Model file for the job. Use its own axes, mm. Face numbers are marked on the shaded views. A direction names the side the tool comes from. Round coordinates to 2 decimals unless told otherwise and drop trailing zeros. Loops run counter-clockwise (first coordinate to the right, second up) from the corner with the lowest first, then second, coordinate; pieces in that order, holes last. Notation, with made-up numbers: M 3,55 L 25,55 A11 ccw 25,71 Z; hole C 34.5,2.5 d6. An arc over 180 degrees is marked long. Use a Markdown table: item, result. Add a question column.
Item 1: Two-plate mould, pull along Z, no slides. Class the marked faces 1, 2, 3 and 4: +Z half, -Z half, draft (parallel to the pull), parting line (faces both ways), or undercut.
Item 2: Pin check, flat tips, straight feed: P1, Ø0.8, axis at x = 14, z = 10.5, coming from the -Y side; P2, Ø10, axis at x = 24.5, y = -14.5, coming from the +Z side; P3, Ø12, axis at x = 4.5, z = 39.5, coming from the +Y side. Stop position of each tip, or through.
Item 3: Tool access for the marked faces 5, 6, 7 and 8: list every direction of +Z, -Z, +X, -X, +Y, -Y with a clear straight run to the whole face (end or side of a thin tool).
Item 4: Saw through at C-C on y = 29. Write the cut outline in (x, z).
Item 5: Saw through at D-D on z = 17.5. Write the cut outline in (x, y).
Item 6: Wall check: L1, parallel to Z at x = 26, y = 15; L2, parallel to X at y = 40, z = 59.7; L3, parallel to Z at x = 7.5, y = -40. Give the ranges that are in metal, low to high. Write a range as from..to.
Item 7: Saw through at A-A on y = -34. Write the cut outline in (x, z).
Item 8: Saw through at B-B on y = -46. Write the cut outline in (x, z).
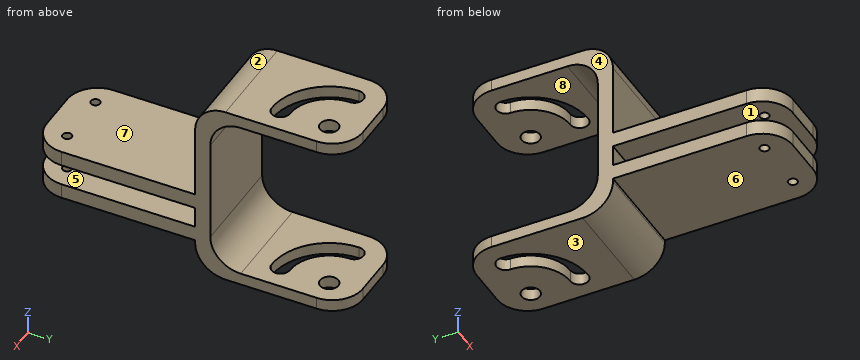
```python
from build123d import *

# Parameters (mm, degrees)
ESBO_O1_W                = 33
ESBO_O1_H                = 50
ESBO_O1_R                = 3
RESSALTO_EXTRUS_O2_DEPTH = 62
ESBO_O3_W                = 33
ESBO_O3_H                = 54
CORTE_EXTRUS_O1_DEPTH    = 45
ESBO_O7_W                = 33
ESBO_O7_H                = 5
RESSALTO_EXTRUS_O3_DEPTH = 54
ESBO_O10_R               = 1.5
CORTE_EXTRUS_O2_DEPTH    = 82.277303105
FILETE1_R                = 10


with BuildPart() as part:
    # Esboço1 → Ressalto-extrusão2 (new body)
    with BuildSketch(Plane.XY):
        with Locations((16.5, 25)):
            Rectangle(ESBO_O1_W, ESBO_O1_H)
        with Locations((25, 40)):
            Circle(ESBO_O1_R, mode=Mode.SUBTRACT)
        with BuildLine():
            ThreePointArc((6, 40), (11.564971157, 26.564971157), (25, 21))
            ThreePointArc((25, 21), (28, 24), (25, 27))
            ThreePointArc((25, 27), (15.807611845, 30.807611845), (12, 40))
            ThreePointArc((12, 40), (9, 43), (6, 40))
        make_face(mode=Mode.SUBTRACT)
    extrude(amount=RESSALTO_EXTRUS_O2_DEPTH)

    # Esboço3 → Corte-extrusão1 (cut)
    with BuildSketch(Plane(origin=(0, 50, 0), x_dir=(1, 0, 0), z_dir=(0, 1, 0))):
        with Locations((16.5, -31)):
            Rectangle(ESBO_O3_W, ESBO_O3_H)
    extrude(amount=-CORTE_EXTRUS_O1_DEPTH, mode=Mode.SUBTRACT)

    # Esboço7 → Ressalto-extrusão3 (add)
    with BuildSketch(Plane.XZ):
        with Locations((16.5, 25.5)):
            Rectangle(ESBO_O7_W, ESBO_O7_H)
        with Locations((16.5, 13.5)):
            Rectangle(ESBO_O7_W, ESBO_O7_H)
    extrude(amount=RESSALTO_EXTRUS_O3_DEPTH)

    # Esboço10 → Corte-extrusão2 (cut, through all)
    with BuildSketch(Plane(origin=(0, 0, 11), x_dir=(-1, 0, 0), z_dir=(0, 0, -1))):
        with Locations((-25.5, -46)):
            Circle(ESBO_O10_R)
        with Locations((-7.5, -46)):
            Circle(ESBO_O10_R)
    extrude(amount=-CORTE_EXTRUS_O2_DEPTH, mode=Mode.SUBTRACT)

    # Filete1
    filete1_edges = [part.edges().sort_by_distance(p)[0] for p in [
        (0, 50, 2),
        (33, 50, 2),
        (16.5, 5, 4),
        (16.5, 5, 58),
        (16.5, 0, 62),
        (16.5, 0, 0),
        (33, -54, 25.5),
        (0, -54, 25.5),
        (33, -54, 13.5),
        (0, -54, 13.5),
        (0, 50, 60),
        (33, 50, 60),
    ]]
    fillet(filete1_edges, radius=FILETE1_R)


solid = part.part
```
Entries:
| question | item | result |
|---|---|---|
| 1 | face 1 | undercut |
| 1 | face 2 | +Z half |
| 1 | face 3 | -Z half |
| 1 | face 4 | draft |
| 2 | P1 | y = 0 |
| 2 | P2 | z = 28 |
| 2 | P3 | y = 5 |
| 3 | face 5 | +X, -X, -Y |
| 3 | face 6 | -Z, +X, -X, -Y |
| 3 | face 7 | +Z, +X, -X, -Y |
| 3 | face 8 | +X, -X, +Y |
| 4 | outline | M 0,0 L 9.51,0 L 9.51,4 L 0,4 Z; M 0,58 L 9.51,58 L 9.51,62 L 0,62 Z; M 18.07,0 L 33,0 L 33,4 L 18.07,4 Z; M 18.07,58 L 33,58 L 33,62 L 18.07,62 Z |
| 5 | outline | M 0,0 L 33,0 L 33,5 L 0,5 Z |
| 6 | L1 | 0..4, 58..62 |
| 6 | L2 | 0..6, 12..22, 28..33 |
| 6 | L3 | 11..16, 23..28 |
| 7 | outline | M 0,11 L 33,11 L 33,16 L 0,16 Z; M 0,23 L 33,23 L 33,28 L 0,28 Z |
| 8 | outline | M 0.2,11 L 6,11 L 6,16 L 0.2,16 Z; M 0.2,23 L 6,23 L 6,28 L 0.2,28 Z; M 9,11 L 24,11 L 24,16 L 9,16 Z; M 9,23 L 24,23 L 24,28 L 9,28 Z; M 27,11 L 32.8,11 L 32.8,16 L 27,16 Z; M 27,23 L 32.8,23 L 32.8,28 L 27,28 Z |
